Verification items for the finished model (mm, model axes). A direction names the side the tool comes from. Give positions to 0.01 mm unless a question says otherwise; leave off trailing zeros. Write each loop counter-clockwise with the first axis right and the second up, starting at its lowest first coordinate (ties: lowest second). Pieces come first, ordered by that corner, then holes. Notation, with made-up numbers: (-8.5, -37.75) -> (39.5, -37.75) arc R30 ccw to (39.5, 0.25) -> close; hole circle Ø1 at (23.25, 38.25). An arc over 180 degrees is marked (long way). Use one line per item in the form item = value. Start each with the question number.
(1) Section check A-A, the plane y = 9. Record the cut outline in (x, z).
(2) Release check for a two-part mould opening along Z. For faces 4 (the face through (-35, 9, 7.442)), 5 (the face through (-35, 14, 6)), 6 (the face through (-35, -10, 21.805)), 7 (the face through (-35, 2, 30.442)) record: pulls with the +Z half, pulls with the -Z half, needs draft (parallel to the pull), parting line crosses it, or undercut.
(3) Section check D-D, the plane z = 23. Record the cut outline in (x, y).
(4) Scan lines: L1, parallel to Z at x = -26.5, y = 10; L2, parallel to Z at x = -41.5, y = -16; L3, parallel to Y at x = -35, z = 40.5. Record each from-to range of solid material in increasing order.
(5) Section check B-B, the plane z = 29.5. Record the cut outline in (x, y), plus the area to 3 significant figures.
(6) Section check C-C, the plane x = -38.25. Record the cut outline in (y, z), plus the area to 3 significant figures.
(7) Depth check by flat-ended pin: pin 1 Ø1.8 at (x, y) = (-27.83, 9) entering from -Z; pin 2 Ø7.5 at (x, z) = (-36.5, 10) entering from +Y; pin 3 Ø1.6 at (y, z) = (-12, 23) entering from +X; pin 4 Ø3 at (x, y) = (-28, -12.5) entering from +Z. Enter the tip coordinate at first touch or a pass-through.
(8) Set-up check for faces 1 (the face through (-41.832, -10, 23)), 2 (the face through (-35, 9, 14.442)), 3 (the face through (-35, 4, 23)): record each of +Z, -Z, +X, -X, +Y, -Y from which the full face is reachable in a straight line by a thin tool's end or side.
from build123d import *

# Parameters (mm, degrees)
SKETCH_2_W          = 22
SKETCH_2_H          = 25
EXTRUDE_1_DEPTH     = 4
SKETCH_3_W          = 22
SKETCH_3_H          = 2
EXTRUDE_2_DEPTH     = 10
SKETCH_4_R          = 1.5
CUT_EXTRUDE_1_DEPTH = 11
SKETCH_5_W          = 14
SKETCH_5_H          = 2
EXTRUDE_3_DEPTH     = 20
SKETCH_6_R          = 2
EXTRUDE_4_DEPTH     = 30


with BuildPart() as part:
    # Эскиз2 → Бобышка-Вытянуть1 (new body)
    with BuildSketch(Plane(origin=(0, 0, 0), x_dir=(1, 0, 0), z_dir=(0, 1, 0))):
        with Locations((-34.831985697, -17.94161698)):
            Rectangle(SKETCH_2_W, SKETCH_2_H)
    extrude(amount=EXTRUDE_1_DEPTH)

    # Эскиз3 → Бобышка-Вытянуть2 (add)
    with BuildSketch(Plane(origin=(0, 4, 0), x_dir=(1, 0, 0), z_dir=(0, 1, 0))):
        with Locations((-34.831985697, -6.44161698)):
            Rectangle(SKETCH_3_W, SKETCH_3_H)
        with Locations((-34.831985697, -15.44161698)):
            Rectangle(SKETCH_3_W, SKETCH_3_H)
    extrude(amount=EXTRUDE_2_DEPTH)

    # Эскиз4 → Вырез-Вытянуть1 (cut)
    with BuildSketch(Plane.XY.offset(16.44161698)):
        with Locations((-41.831985697, 9)):
            Circle(SKETCH_4_R)
        with Locations((-27.831985697, 9)):
            Circle(SKETCH_4_R)
    extrude(amount=-CUT_EXTRUDE_1_DEPTH, mode=Mode.SUBTRACT)

    # Эскиз5 → Бобышка-Вытянуть3 (add)
    with BuildSketch(Plane.XZ):
        with Locations((-34.831985697, 22.805333719)):
            Rectangle(SKETCH_5_W, SKETCH_5_H)
    extrude(amount=EXTRUDE_3_DEPTH)

    # Эскиз6 → Бобышка-Вытянуть4 (add)
    with BuildSketch(Plane.XY.offset(23.805333719)):
        with Locations(Location((-34.831985697, -10, 0), (0, 0, 180))):
            Circle(SKETCH_6_R)
    extrude(amount=EXTRUDE_4_DEPTH)


solid = part.part
Completed:
q1.outline = (-45.83, 5.44) -> (-43.33, 5.44) -> (-43.33, 7.44) -> (-45.83, 7.44) -> close; (-45.83, 14.44) -> (-43.33, 14.44) -> (-43.33, 16.44) -> (-45.83, 16.44) -> close; (-40.33, 5.44) -> (-29.33, 5.44) -> (-29.33, 7.44) -> (-40.33, 7.44) -> close; (-40.33, 14.44) -> (-29.33, 14.44) -> (-29.33, 16.44) -> (-40.33, 16.44) -> close; (-26.33, 5.44) -> (-23.83, 5.44) -> (-23.83, 7.44) -> (-26.33, 7.44) -> close; (-26.33, 14.44) -> (-23.83, 14.44) -> (-23.83, 16.44) -> (-26.33, 16.44) -> close
q2.face_4 = undercut
q2.face_5 = needs draft
q2.face_6 = pulls with the -Z half
q2.face_7 = pulls with the +Z half
q3.outline = (-45.83, 0) -> (-41.83, 0) -> (-41.83, -20) -> (-27.83, -20) -> (-27.83, 0) -> (-23.83, 0) -> (-23.83, 4) -> (-45.83, 4) -> close
q4.L1 = 5.44 to 7.44, 14.44 to 16.44
q4.L2 = 21.81 to 23.81
q4.L3 = -11.99 to -8.01
q5.outline = (-45.83, 0) -> (-23.83, 0) -> (-23.83, 4) -> (-45.83, 4) -> close; circle Ø4 at (-34.83, -10)
q5.area = 101 mm²
q6.outline = (-20, 21.81) -> (0, 21.81) -> (0, 5.44) -> (14, 5.44) -> (14, 7.44) -> (4, 7.44) -> (4, 14.44) -> (14, 14.44) -> (14, 16.44) -> (4, 16.44) -> (4, 30.44) -> (0, 30.44) -> (0, 23.81) -> (-20, 23.81) -> close
q6.area = 180 mm²
q7.pin_1 = through
q7.pin_2 = 14
q7.pin_3 = -27.83
q7.pin_4 = 23.81
q8.face_1 = +Z, -Z, -X, -Y
q8.face_2 = +X, -X, +Y
q8.face_3 = +Z, +X, -X, +Y
